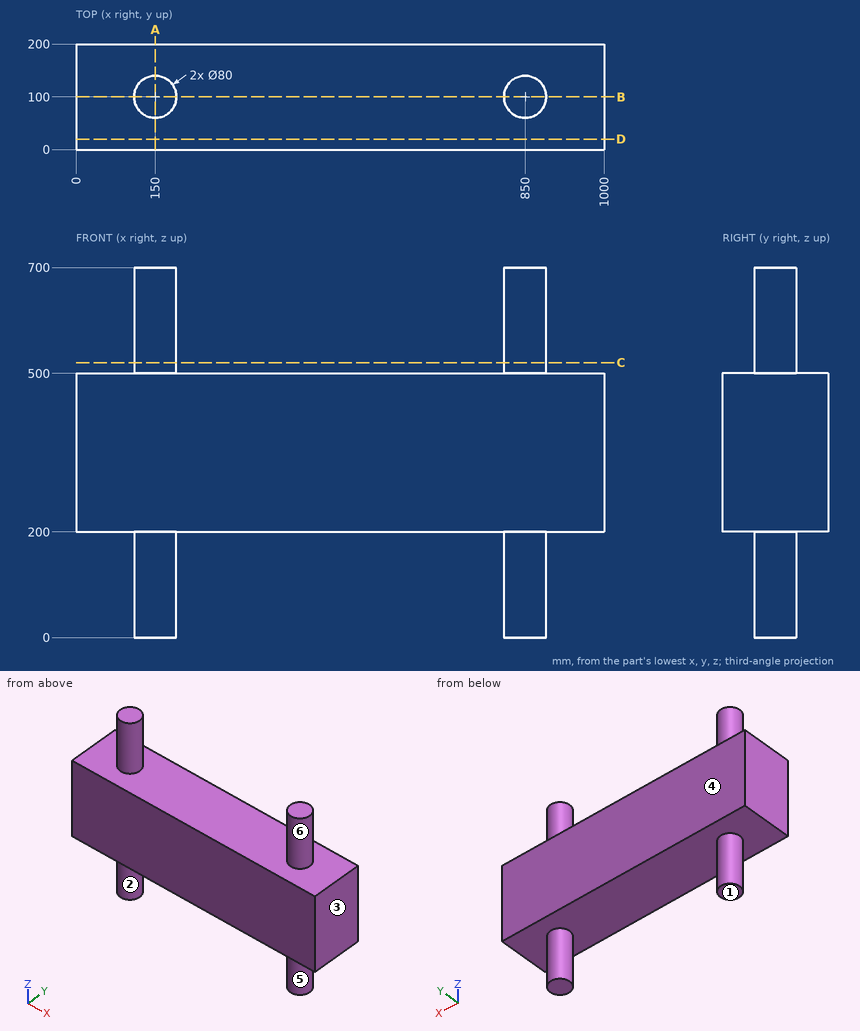
Answer from the drawing. Dimensions are ordinates in mm from the lowest x, y and z of the part. A direction names the side the tool comes from. Give positions to 0.01 mm unless a question says otherwise; leave off trailing zeros. Loops run counter-clockwise (first coordinate to the right, second up) from the corner with the lowest first, then second, coordinate; pieces in that order, holes last. Notation, with made-up numbers: (-22.5, 31) -> (-14.5, 31) arc R12 cw to (-14.5, 41) -> close; hole circle Ø4 at (-33.5, -9.5). An arc over 180 degrees is marked (long way). Answer as CSV lines item,"result".
Item 1: Find section A-A on x = 150. Give the vertices of the cut face in (y, z), plus the area to 3 significant figures.
Returned:
outline,"(0, 200) -> (60, 200) -> (60, 0) -> (140, 0) -> (140, 200) -> (200, 200) -> (200, 500) -> (140, 500) -> (140, 700) -> (60, 700) -> (60, 500) -> (0, 500) -> close"
area,"92,000 mm²"
Item 2: Find section B-B on y = 100. Give the vertices of the cut face in (x, z).
Returned:
outline,"(0, 200) -> (110, 200) -> (110, 0) -> (190, 0) -> (190, 200) -> (810, 200) -> (810, 0) -> (890, 0) -> (890, 200) -> (1000, 200) -> (1000, 500) -> (890, 500) -> (890, 700) -> (810, 700) -> (810, 500) -> (190, 500) -> (190, 700) -> (110, 700) -> (110, 500) -> (0, 500) -> close"
Item 3: Consider line 1 (Z direction, x = 166.5, y = 47.5); line 2 (X direction, y = 64, z = 563); line 3 (X direction, y = 86, z = 114). Determine where each line is inside the solid, lowest interval first. Write a range as [from, to].
Returned:
line 1,"z = [200, 500]"
line 2,"x = [132.56, 167.44], [832.56, 867.44]"
line 3,"x = [112.53, 187.47], [812.53, 887.47]"
Item 4: Determine the mould class of the marked faces 1, 2 and 3 for opening direction X: +X half, -X half, draft (parallel to the pull), parting line (faces both ways), or undercut.
Returned:
face 1,"draft"
face 2,"undercut"
face 3,"+X half"
Item 5: Each of these flat-tipped pins is pushed along its axis until it touches: pin 1 (8 mm diameter, centred on x = 234, y = 125.5, fed in from +Z); pin 2 (2 mm diameter, centred on x = 725.5, y = 108.5, fed in from -Z); pin 3 (5 mm diameter, centred on x = 835, z = 593.5, fed in from -Y). Where does it stop, or does it pass through?
Returned:
pin 1,"stops at z = 500"
pin 2,"stops at z = 200"
pin 3,"stops at y = 62"
Item 6: For the marked faces 4, 5 and 6, determine the directions among +Z, -Z, +X, -X, +Y, -Y from which every point of the face is accessible in a straight line to the end or side of a thin tool.
Returned:
face 4,"+Z, -Z, +X, -X, +Y"
face 5,"-Z"
face 6,"+Z"
Item 7: Find section D-D on y = 20. Give the vertices of the cut face in (x, z), plus the area to 3 significant figures.
Returned:
outline,"(0, 200) -> (1000, 200) -> (1000, 500) -> (0, 500) -> close"
area,"300,000 mm²"
Item 8: Find section C-C on z = 520.5. Give the vertices of the cut face in (x, y), plus the area to 3 significant figures.
Returned:
outline,"circle Ø80 at (150, 100); circle Ø80 at (850, 100)"
area,"10,100 mm²"
